Input: part model. Units: mm. Frame: model coordinates. Round coordinates to 2 decimals unless told otherwise and drop trailing zeros. Order: outer loops, then holes, each group sorted by start corner. A loop starts at its lowest first (then second) coordinate and runs counter-clockwise, first axis right, second up. Notation, with made-up numbers: (-9.5, 88) -> (47.5, 88) arc R31 cw to (47.5, 122) -> close; hole circle Ø4 at (27, 86.25). An arc over 180 degrees is marked (long way). Use a Markdown table: item, result.
from build123d import *

# Parameters (mm, degrees)
BOSS_EXTRU_1_DEPTH = 2
CONG_1_R           = 2


with BuildPart() as part:
    # Esquisse1 → Boss.-Extru.1 (new body)
    with BuildSketch(Plane.XY):
        with BuildLine():
            Line((-36, 84), (56, 84))
            Line((56, 84), (56, -23))
            Line((56, -23), (38.678159212, -23))
            ThreePointArc((38.678159212, -23), (25.035836998, 37.392604427), (-36, 27))
            Line((-36, 27), (-36, 84))
        make_face()
    extrude(amount=BOSS_EXTRU_1_DEPTH)

    # Congé1
    cong_1_edges = [part.edges().sort_by_distance(p)[0] for p in [
        (38.678159212, -23, 1),
        (-36, 27, 1),
    ]]
    fillet(cong_1_edges, radius=CONG_1_R)


solid = part.part
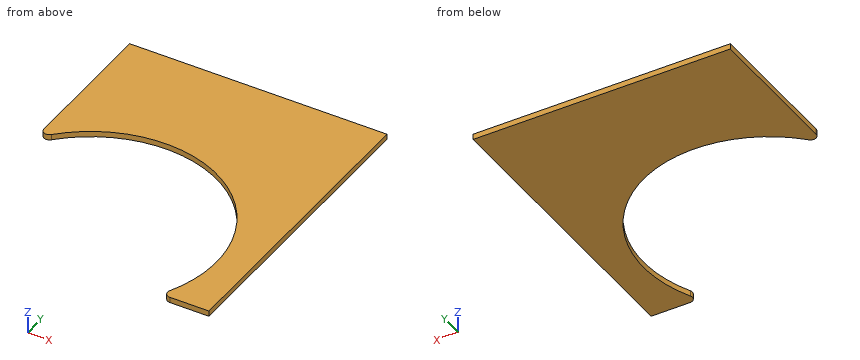
1) Cut plane B-B on y = 9.5. Return loops of the section in (x, z), and give its area (3 significant figures).
Answer key:
| item | result |
|---|---|
| outline | (43.99, 0) -> (56, 0) -> (56, 2) -> (43.99, 2) -> close |
| area | 24.0 mm^2 |
2) Cut plane C-C on x = -14. Return loops of the section in (y, z).
Answer key:
| item | result |
|---|---|
| outline | (42.77, 0) -> (84, 0) -> (84, 2) -> (42.77, 2) -> close |
3) Ray query, probe 1 along X at (y, z) = (-1, 1.45); probe 2 along X at (y, z) = (40, 0.3); probe 3 along X at (y, z) = (31, 0.5). Return the intervals inside material, ascending.
Answer key:
| item | result |
|---|---|
| probe 1 | x = 44.99 to 56 |
| probe 2 | x = -36 to -20.62, 20.62 to 56 |
| probe 3 | x = -35.38 to -32.62, 32.62 to 56 |
4) Cut plane A-A on z = 1.5. Return loops of the section in (x, y).
Answer key:
| item | result |
|---|---|
| outline | (-36, 32.45) arc R2 ccw to (-32.55, 31.07) arc R45 cw to (40.26, -20.11) arc R2 ccw to (42.05, -23) -> (56, -23) -> (56, 84) -> (-36, 84) -> close |
